Geometry: final body of the model. Coordinates: model frame, mm. Give positions to 0.01 mm unless a question says otherwise; leave off trailing zeros. Write each loop counter-clockwise with the first axis right and the second up, starting at its lowest first coordinate (ties: lowest second). Pieces come first, ordered by that corner, then holes. Notation, with made-up numbers: (60.5, 50) - (94.5, 50) arc R3 cw to (94.5, 55) - close; hole circle Ø2 at (43.25, 35). An arc over 180 degrees is marked (long way). Return JSON: item names as keys, results as strings.
from build123d import *

# Parameters (mm, degrees)
SKETCH1_R           = 1.1811
RODEND_DEPTH        = 12.7
SKETCH4_R           = 1.1811
REVOLVE1_ANGLE      = 90
SKETCH5_R           = 1.1811
BOSS_EXTRUDE1_DEPTH = 127


with BuildPart() as part:
    # Sketch1 → RodEnd (new body)
    with BuildSketch(Plane.XY):
        Circle(SKETCH1_R)
    extrude(amount=-RODEND_DEPTH)

    # Sketch4 → Revolve1 (revolve)
    with BuildSketch(Plane(origin=(0, 0, -12.7), x_dir=(-1, 0, 0), z_dir=(0, 0, -1))):
        with Locations(Location((0, 0, 0), (0, 0, 180))):
            Circle(SKETCH4_R)
    revolve(axis=Axis((-6.35, 0, -12.7), (0, 1, 0)), revolution_arc=REVOLVE1_ANGLE)

    # Sketch5 → Boss-Extrude1 (add)
    with BuildSketch(Plane.ZY.offset(6.35)):
        with Locations(Location((-19.05, 0, 0), (0, 0, 180))):
            Circle(SKETCH5_R)
    extrude(amount=BOSS_EXTRUDE1_DEPTH)


solid = part.part
Q1. Section query C-C, the plane x = -91. Return the cut outline in (y, z).
Answer key:
{"outline": "circle Ø2.36 at (0, -19.05)"}
Q2. Mould query, pull axis X, two halves, no side actions, for faces 1 (the cylindrical face through (0.63, 1, -6.26)), 2 (the flat face through (-133.35, 0, -19)), 3 (the flat face through (0, 0, 0)). Classes: pulls with the +X half, pulls with the -X half, needs draft (parallel to the pull), parting line crosses it, or undercut.
Answer key:
{"face 1": "parting line crosses it", "face 2": "pulls with the -X half", "face 3": "needs draft"}
Q3. Material intervals for probe 1 along X at (y, z) = (0.2, -1.75); probe 2 along Z at (x, y) = (-26, 0.05); probe 3 along Z at (x, y) = (-69, 0.8), sorted ascending. Write a range as [from, to].
Answer key:
{"probe 1": "x = [-1.16, 1.16]", "probe 2": "z = [-20.23, -17.87]", "probe 3": "z = [-19.92, -18.18]"}
Q4. Section query B-B, the plane z = -10.5. Return the cut outline in (x, y), plus the area to 3 significant figures.
Answer key:
{"outline": "circle Ø2.36 at (0, 0)", "area": "4.38 mm^2"}
Q5. Pin query (flat end, axial travel): P1, Ø1, axis at y = -0.5, z = -11.5, coming from the +X side; P2, Ø12, axis at x = -28, z = -12.5, coming from the +Y side. Return the tip coordinate at first contact, or that it passes through.
Answer key:
{"P1": "stops at x = 1.18", "P2": "stops at y = 1.05"}
Q6. Section query A-A, the plane y = 0. Return the cut outline in (x, z).
Answer key:
{"outline": "(-133.35, -20.23) - (-6.35, -20.23) arc R7.53 ccw to (1.18, -12.7) - (1.18, 0) - (-1.18, 0) - (-1.18, -12.7) arc R5.17 cw to (-6.35, -17.87) - (-133.35, -17.87) - close"}
